Job drawing, mm, ordinate dimensions from the low corner. One solid piece. Round coordinates to 2 decimals unless told otherwise and drop trailing zeros. Write each loop counter-clockwise with the first axis right and the second up, starting at its lowest first coordinate (ties: lowest second). Pieces come first, ordered by that corner, then holes.
1) Saw through at B-B on z = 1.3. Write the cut outline in (x, y).
2) Drill centre lines: L1, parallel to Y at x = 21.5, z = 0.7; L2, parallel to X at y = 13.75, z = 1.2. Where is each one in solid material? Low to high.
3) Saw through at A-A on y = 10. Write the cut outline in (x, z).
4) Saw through at C-C on x = 22. Write the cut outline in (y, z).
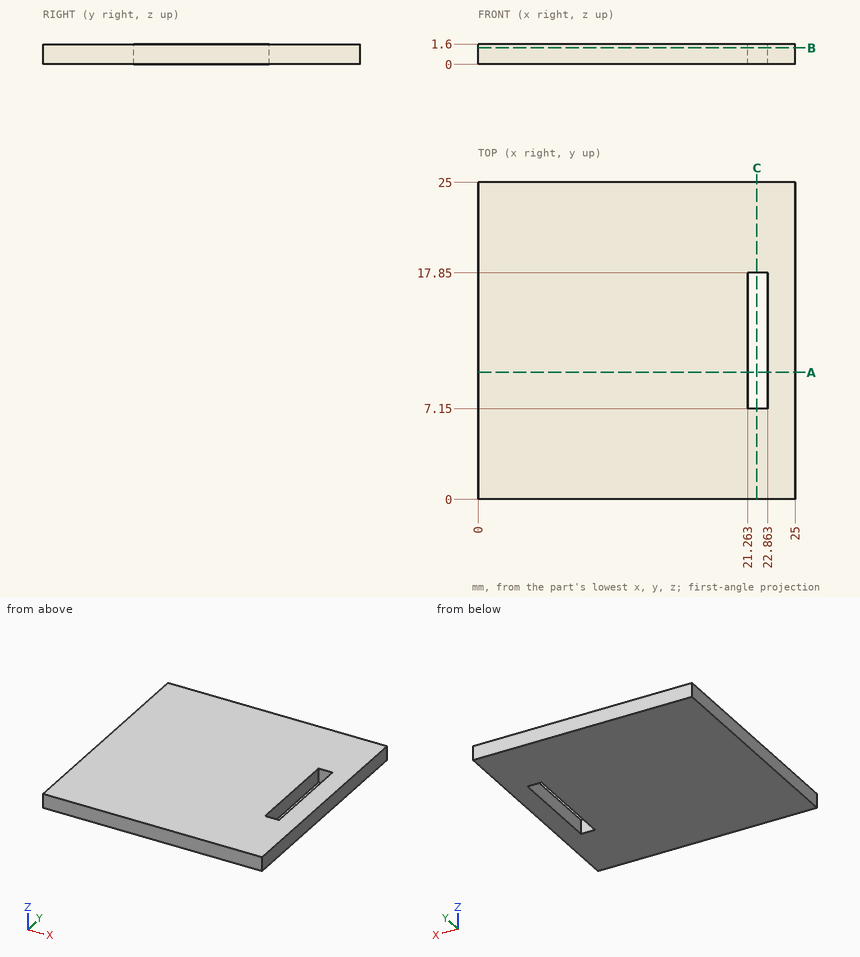
Completed:
1. outline: (0, 0) - (25, 0) - (25, 25) - (0, 25) - close; hole (21.26, 7.15) - (22.86, 7.15) - (22.86, 17.85) - (21.26, 17.85) - close
2. L1: y = 0 to 7.15, 17.85 to 25
2. L2: x = 0 to 21.26, 22.86 to 25
3. outline: (0, 0) - (21.26, 0) - (21.26, 1.6) - (0, 1.6) - close; (22.86, 0) - (25, 0) - (25, 1.6) - (22.86, 1.6) - close
4. outline: (0, 0) - (7.15, 0) - (7.15, 1.6) - (0, 1.6) - close; (17.85, 0) - (25, 0) - (25, 1.6) - (17.85, 1.6) - close
